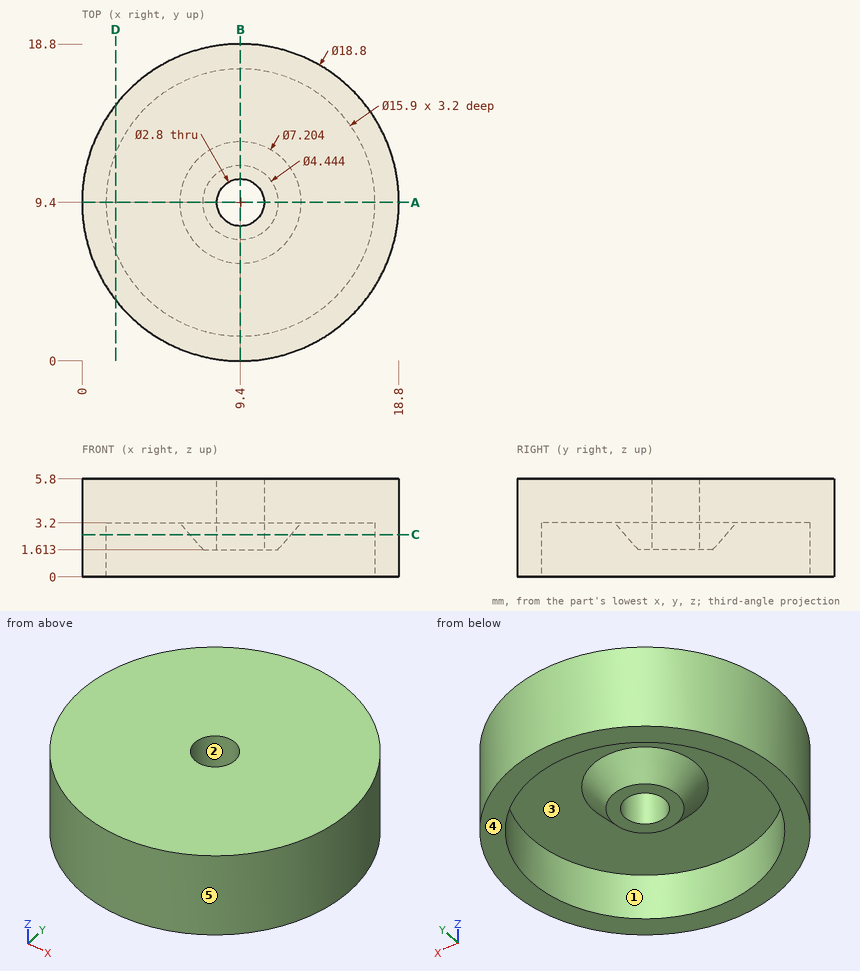
Job drawing, mm, ordinate dimensions from the low corner. One solid piece. A direction names the side the tool comes from. Round coordinates to 2 decimals unless told otherwise and drop trailing zeros. Loops run counter-clockwise (first coordinate to the right, second up) from the corner with the lowest first, then second, coordinate; pieces in that order, holes last. Notation, with made-up numbers: (-19, 22) -> (36, 22) arc R11 cw to (36, 40) -> close; hole circle Ø3 at (2.25, -25.75). An arc over 180 degrees is marked (long way). One line per item, written item: value. Start each with the question number.
Q1. Probe line 1 along Y through (x, z) = (9.4, 4.55); line 2 along Y through (x, z) = (9.25, 0.45); line 3 along X through (y, z) = (2.25, 0.9) (1 decimal). List the from-to ranges inside material, lowest first.
Q2. 3-axis set-ups, long thin cutter, end or side, ignore diameter. For the marked faces 1 and 2: which of +Z, -Z, +X, -X, +Y, -Y reach the whole face in a straight line?
Q3. Cut at A-A on y = 9.4. List the corners of the cut face in (x, z).
Q4. Drop flat-ended pins along their axis: pin 1 Ø1 at (x, y) = (7.5, 13) entering from -Z (1 decimal); pin 2 Ø5 at (x, y) = (10.5, 10) entering from -Z. Give the stop position or say it passes through.
Q5. Cut at C-C on z = 2.5. List the corners of the cut face in (x, y), plus the area to 3 significant figures.
Q6. Cut at D-D on x = 2. List the corners of the cut face in (y, z) (1 decimal).
Q7. Two-plate mould, pull along Y, no slides. Class the marked faces 3, 4 and 5: released by +Y, released by -Y, zero draft, split by the parting line, or undercut.
Computed:
1. line 1: 0 to 8, 10.8 to 18.8
1. line 2: 0 to 1.45, 17.35 to 18.8
1. line 3: 3.3 to 5.9, 12.9 to 15.5
2. face 1: -Z
2. face 2: +Z, -Z
3. outline: (0, 0) -> (1.45, 0) -> (1.45, 3.2) -> (5.8, 3.2) -> (7.18, 1.61) -> (8, 1.61) -> (8, 5.8) -> (0, 5.8) -> close; (10.8, 1.61) -> (11.62, 1.61) -> (13, 3.2) -> (17.35, 3.2) -> (17.35, 0) -> (18.8, 0) -> (18.8, 5.8) -> (10.8, 5.8) -> close
4. pin 1: z = 3.2
4. pin 2: z = 1.61
5. outline: circle Ø18.8 at (9.4, 9.4); circle Ø5.99 at (9.4, 9.4); hole circle Ø15.9 at (9.4, 9.4); hole circle Ø2.8 at (9.4, 9.4)
5. area: 101 mm²
6. outline: (3.6, 0) -> (6.5, 0) -> (6.5, 3.2) -> (12.3, 3.2) -> (12.3, 0) -> (15.2, 0) -> (15.2, 5.8) -> (3.6, 5.8) -> close
7. face 3: undercut
7. face 4: zero draft
7. face 5: split by the parting line
